Autodesk Inventor part; units mm, degrees
ref_plane "YZ Plane" through (0, 0, 0) normal (1, 0, 0) x (0, 1, 0)
ref_plane "XZ Plane" through (0, 0, 0) normal (0, 1, 0) x (-1, 0, 0)
ref_plane "XY Plane" through (0, 0, 0) normal (0, 0, 1) x (1, 0, 0)
sketch "Sketch1" plane through (0, 0, 0) normal (0, 1, 0) x (-1, 0, 0)
  line L0 (0, 0) -> (0, -76.2)
  line L1 (0, -76.2) -> (35.09, -76.2)
  line L2 (35.09, -76.2) -> (35.09, 0)
  line L3 (35.09, 0) -> (0, 0)
  line L4 (8.89, 0) -> (8.89, -76.2)
  line L5 (9.69, 0) -> (9.69, -76.2)
  dimension "d1" = 76.2
  dimension "d2" = 35.09
  dimension "d3" = 8.89
  dimension "d4" = 0.8
extrude "Extrusion1" add sketch "Sketch1" along normal blind 6.35
extrude "Extrusion2" add sketch "Sketch1" along normal blind 25.4 contours L3 L4 L1 L0
extrude "Extrusion3" add sketch "Sketch1" along normal blind 25.4 contours L3 L2 L1 L5
sketch "Sketch2" plane through (0, 0, 0) normal (1, 0, 0) x (0, 0, -1)
  line L0 (0, 0) -> (0, 25.4)
  line L1 (0, 12.7) -> (76.2, 12.7)
  line L2 (76.2, 6.35) -> (76.2, 25.4)
  circle A0 centre (7.62, 12.7) radius 1.716
  line L3 (15.24, 12.7) -> (34.544, 12.7)
  line L4 (34.544, 12.7) -> (34.544, 13.716)
  line L5 (34.544, 13.716) -> (15.24, 13.716)
  line L6 (15.24, 13.716) -> (15.24, 12.7)
  line L7 (39.624, 12.7) -> (52.578, 12.7)
  line L8 (52.578, 12.7) -> (52.578, 13.716)
  line L9 (52.578, 13.716) -> (39.624, 13.716)
  line L10 (39.624, 13.716) -> (39.624, 12.7)
  circle A1 centre (57.658, 12.7) radius 1.0033
  circle A2 centre (67.4281, 12.7) radius 4.7752
  point P0 (15.24, 13.208)
  point P1 (39.624, 13.208)
  point P2 (34.544, 13.208)
  point P3 (52.578, 13.208)
  dimension "d13" = 19.304
  dimension "d14" = 1.016
  dimension "d15" = 12.954
  dimension "d16" = 1.016
  dimension "d19" = 2.0066
  dimension "d22" = 7.62
  dimension "d23" = 7.62
  dimension "d24" = 5.08
  dimension "d25" = 5.08
  dimension "d26" = 9.5504
extrude "Extrusion4" cut sketch "Sketch2" against normal blind 28.486 contours A0 L1 | L1 A0
extrude "Extrusion5" cut sketch "Sketch2" against normal blind 27.978 contours L10 L9 L8 L1 | L6 L5 L4 L1
extrude "Extrusion6" cut sketch "Sketch2" against normal blind 18.58 contours A1 L1 | L1 A1
extrude "Extrusion7" cut sketch "Sketch2" against normal blind 11.2394 contours A2 L1 | L1 A2
properties part number "Cutting Jig"
For this review, take the finished solid that the model builds, in its own axes (mm). A direction names the side the tool comes from. Round coordinates to 2 decimals unless told otherwise and drop trailing zeros. Write each loop counter-clockwise with the first axis right and the second up, starting at its lowest first coordinate (ties: lowest second). Pieces come first, ordered by that corner, then holes. Notation, with made-up numbers: M 37,-3 L 94,-3 A16 ccw 94,20 Z; hole C 55.5,2 d7. An arc over 180 degrees is marked long. One line per item, written item: value. Start each with the question number.
(1) We need section D-D (z = -24). Give the boundary of the cut face in (x, y), and give its area (3 significant figures).
(2) We need section A-A (z = -7.62). Give the boundary of the cut face in (x, y), and give its area (3 significant figures).
(3) We need section C-C (x = -3). Give the boundary of the cut face in (y, z).
(4) Insertion check: pin 1 (1.8 mm diameter, centred on y = 12.7, z = -57.658, fed in from +X); pin 2 (10 mm diameter, centred on x = -27.5, z = -20, fed in from -Y); pin 3 (0.5 mm diameter, centred on y = 13, z = -44.5, fed in from +X). Each pin has a flat end and moves straight along its axis. Give the tip position at first contact, or say it passes through.
(5) We need section B-B (x = -12.5). Give the boundary of the cut face in (y, z).
(6) Machinability: for faces 1 (the flat face through (-8.89, 16, -38)), 2 (the flat face through (-18.58, 13, -58)), 3 (the flat face through (-22, 25.4, -38)), which of the approach directions +Z, -Z, +X, -X, +Y, -Y give a long, thin tool a straight path to every point of the face, cutting with its end or side? Answer none if there is none.
(7) The part is to be moulded in two halves that separate along X. For faces 4 (the flat face through (-11.239, 13, -67)), 5 (the cylindrical face through (-4.383, 12.91, -62.658)), 6 (the flat face through (-9.69, 16, -38)), say which applies: released by +X, released by -X, zero draft, split by the parting line, or undercut.
(8) Wall thickness on line 1 (X direction, y = 20.25, z = -6.5); line 2 (Y direction, x = -10.5, z = -34.5); line 3 (Z direction, x = -2, y = 16): over which ranges is each line inside the solid? List them lowest first.
Result:
1. outline: M -35.09,0 L 0,0 L 0,12.7 L -8.89,12.7 L -8.89,6.35 L -9.69,6.35 L -9.69,12.7 L -27.98,12.7 L -27.98,13.72 L -9.69,13.72 L -9.69,25.4 L -35.09,25.4 Z; M -8.89,13.72 L 0,13.72 L 0,25.4 L -8.89,25.4 Z
1. area: 848 mm²
2. outline: M -35.09,0 L 0,0 L 0,10.98 L -8.89,10.98 L -8.89,6.35 L -9.69,6.35 L -9.69,10.98 L -28.49,10.98 L -28.49,14.42 L -9.69,14.42 L -9.69,25.4 L -35.09,25.4 Z; M -8.89,14.42 L 0,14.42 L 0,25.4 L -8.89,25.4 Z
2. area: 781 mm²
3. outline: M 0,-76.2 L 25.4,-76.2 L 25.4,0 L 0,0 Z; hole C 12.7,-67.43 d9.55; hole C 12.7,-7.62 d3.43; hole C 12.7,-57.66 d2.01; hole M 12.7,-52.58 L 13.72,-52.58 L 13.72,-39.62 L 12.7,-39.62 Z; hole M 12.7,-34.54 L 13.72,-34.54 L 13.72,-15.24 L 12.7,-15.24 Z
4. pin 1: x = -18.58
4. pin 2: y = 0
4. pin 3: x = -27.98
5. outline: M 0,-76.2 L 25.4,-76.2 L 25.4,0 L 0,0 Z; hole C 12.7,-7.62 d3.43; hole C 12.7,-57.66 d2.01; hole M 12.7,-52.58 L 13.72,-52.58 L 13.72,-39.62 L 12.7,-39.62 Z; hole M 12.7,-34.54 L 13.72,-34.54 L 13.72,-15.24 L 12.7,-15.24 Z
6. face 1: +Z, -Z, +Y
6. face 2: +X
6. face 3: +Z, -Z, +X, -X, +Y
7. face 4: released by +X
7. face 5: zero draft
7. face 6: undercut
8. line 1: -35.09 to -9.69, -8.89 to 0
8. line 2: 0 to 12.7, 13.72 to 25.4
8. line 3: -76.2 to -70.88, -63.98 to 0
